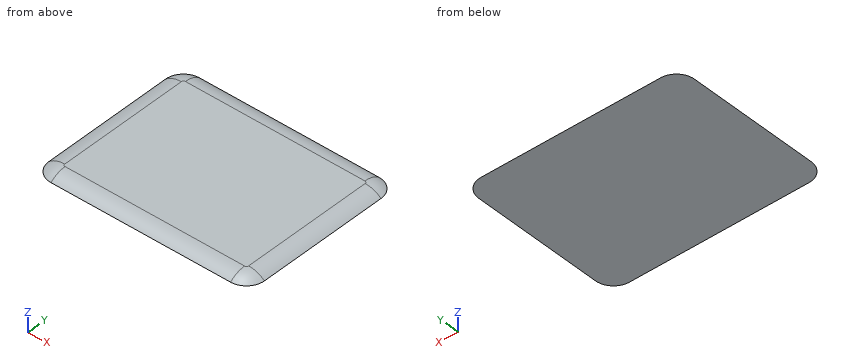
```python
from build123d import *

# Parameters (mm, degrees)
F1_DEPTH     = 1.27
F2_T1_DEPTH  = 27.94
F2_T3_DEPTH  = 38.1
F2_T6_ANGLE  = 90
F2_T8_ANGLE  = 90
F2_T10_ANGLE = 90
F2_T12_ANGLE = 90


# Not quite as in the source:
# - a fillet or chamfer that OpenCascade refuses, or shapes differently, is made with other operations: its cross-section is extruded or revolved along the edge and cut away or added


with BuildPart() as f1:
    # F0 (on Top) → F1 (new body)
    with BuildSketch(Plane.XY):
        with BuildLine():
            ThreePointArc((22.86, 13.97), (21.7440768363, 16.6640768363), (19.05, 17.78))
            Line((19.05, 17.78), (-19.05, 17.78))
            ThreePointArc((-19.05, 17.78), (-21.7440768363, 16.6640768363), (-22.86, 13.97))
            Line((-22.86, 13.97), (-22.86, -13.97))
            ThreePointArc((-22.86, -13.97), (-21.7440768363, -16.6640768363), (-19.05, -17.78))
            Line((-19.05, -17.78), (19.05, -17.78))
            ThreePointArc((19.05, -17.78), (21.7440768363, -16.6640768363), (22.86, -13.97))
            Line((22.86, -13.97), (22.86, 13.97))
        make_face()
    extrude(amount=F1_DEPTH)

    # F2: fillet of radius 5.08 on 1 edges, made by hand

    # F2_s2 → F2_t1 (cut)
    with BuildSketch(Plane.XZ.offset(-13.97)):
        with BuildLine():
            ThreePointArc((-22.86, 0), (-21.2959470592, 0.9419048812), (-19.4998958349, 1.27))
            Line((-19.4998958349, 1.27), (-22.86, 1.27))
            Line((-22.86, 1.27), (-22.86, 0))
        make_face()
        with BuildLine():
            ThreePointArc((22.86, 0), (21.2959470592, 0.9419048812), (19.4998958349, 1.27))
            Line((19.4998958349, 1.27), (22.86, 1.27))
            Line((22.86, 1.27), (22.86, 0))
        make_face()
    extrude(amount=F2_T1_DEPTH, mode=Mode.SUBTRACT)

    # F2_s4 → F2_t3 (cut)
    with BuildSketch(Plane.YZ.offset(-19.05)):
        with BuildLine():
            ThreePointArc((-17.78, 0), (-16.2159470592, 0.9419048812), (-14.4198958349, 1.27))
            Line((-14.4198958349, 1.27), (-17.78, 1.27))
            Line((-17.78, 1.27), (-17.78, 0))
        make_face()
        with BuildLine():
            ThreePointArc((17.78, 0), (16.2159470592, 0.9419048812), (14.4198958349, 1.27))
            Line((14.4198958349, 1.27), (17.78, 1.27))
            Line((17.78, 1.27), (17.78, 0))
        make_face()
    extrude(amount=F2_T3_DEPTH, mode=Mode.SUBTRACT)

    # F2_s5 → F2_t6 (revolve, cut)
    with BuildSketch(Plane.YZ.offset(-19.05)):
        with BuildLine():
            ThreePointArc((17.78, 0), (16.2159470592, 0.9419048812), (14.4198958349, 1.27))
            Line((14.4198958349, 1.27), (17.78, 1.27))
            Line((17.78, 1.27), (17.78, 0))
        make_face()
    revolve(axis=Axis((-19.05, 13.97, 1.27), (0, 0, 1)), revolution_arc=F2_T6_ANGLE, mode=Mode.SUBTRACT)

    # F2_s7 → F2_t8 (revolve, cut)
    with BuildSketch(Plane.XZ.offset(13.97)):
        with BuildLine():
            ThreePointArc((-22.86, 0), (-21.2959470592, 0.9419048812), (-19.4998958349, 1.27))
            Line((-19.4998958349, 1.27), (-22.86, 1.27))
            Line((-22.86, 1.27), (-22.86, 0))
        make_face()
    revolve(axis=Axis((-19.05, -13.97, 1.27), (0, 0, 1)), revolution_arc=F2_T8_ANGLE, mode=Mode.SUBTRACT)

    # F2_s9 → F2_t10 (revolve, cut)
    with BuildSketch(Plane.YZ.offset(19.05)):
        with BuildLine():
            ThreePointArc((-17.78, 0), (-16.2159470592, 0.9419048812), (-14.4198958349, 1.27))
            Line((-14.4198958349, 1.27), (-17.78, 1.27))
            Line((-17.78, 1.27), (-17.78, 0))
        make_face()
    revolve(axis=Axis((19.05, -13.97, 1.27), (0, 0, 1)), revolution_arc=F2_T10_ANGLE, mode=Mode.SUBTRACT)

    # F2_s11 → F2_t12 (revolve, cut)
    with BuildSketch(Plane.XZ.offset(-13.97)):
        with BuildLine():
            ThreePointArc((22.86, 0), (21.2959470592, 0.9419048812), (19.4998958349, 1.27))
            Line((19.4998958349, 1.27), (22.86, 1.27))
            Line((22.86, 1.27), (22.86, 0))
        make_face()
    revolve(axis=Axis((19.05, 13.97, 1.27), (0, 0, 1)), revolution_arc=F2_T12_ANGLE, mode=Mode.SUBTRACT)


solid = f1.part
```
Geometry: final body of the model. Coordinates: model frame, mm. Coordinates: 2 decimals unless noted, no trailing zeros. Order: outer loops, then holes, each group sorted by start corner. A loop starts at its lowest first (then second) coordinate and runs counter-clockwise, first axis right, second up. Notation, with made-up numbers: M 6.5,-18 L 37.5,-18 A24 cw 37.5,-1 Z; hole C -37.75,54.5 d10. An arc over 180 degrees is marked long. Answer in a Markdown table with one row per item. Add a question column.
Q1. Section query A-A on y = 3.5. Return the cut outline in (x, z).
Q2. Section query B-B on x = -14.5. Return the cut outline in (y, z), and give its area (3 significant figures).
Q3. Line query: L1, parallel to Z at x = -18.5, y = 14.5; L2, parallel to Y at x = -18.5, z = 0.2; L3, parallel to Y at x = 15.5, z = 0.85. Output: solid intervals per line, ascending.
Completed:
| question | item | result |
|---|---|---|
| 1 | outline | M -22.86,0 L 22.86,0 A5.08 ccw 19.5,1.27 L -19.5,1.27 A5.08 ccw Z |
| 2 | outline | M -17.78,0 L 17.78,0 A5.08 ccw 14.42,1.27 L -14.42,1.27 A5.08 ccw Z |
| 2 | area | 42.5 mm2 |
| 3 | L1 | z = 0 to 1.27 |
| 3 | L2 | y = -17.54 to 17.54 |
| 3 | L3 | y = -16.44 to 16.44 |
